Here's how the part is built. I have some questions about the finished solid (model axes, mm). Face numbers are marked on the shaded views. A direction names the side the tool comes from. Round coordinates to 2 decimals unless told otherwise and drop trailing zeros. Loops run counter-clockwise (first coordinate to the right, second up) from the corner with the lowest first, then second, coordinate; pieces in that order, holes last. Notation, with made-up numbers: M 69,11 L 106,11 A19 cw 106,30 Z; hole C -11.5,32.5 d6. An arc over 180 degrees is marked long. Answer as a JSON object with one key per item and string values.
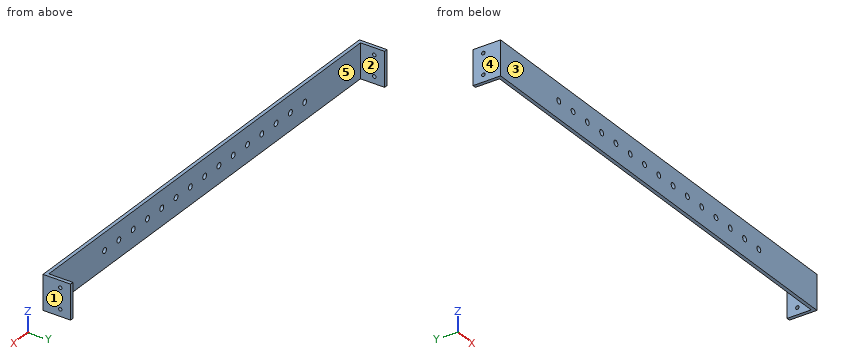
from build123d import *

# Parameters (mm, degrees)
F1_DEPTH      = 25
F2_R          = 4
F3_DEPTH      = 25
F4_R          = 2.5
F5_DEPTH      = 332.001
F5_DEPTH_BACK = 332.001


with BuildPart() as f1:
    # F0 (on Top) → F1 (new body, symmetric)
    with BuildSketch(Plane.XY):
        Polygon((-332, 0), (0, 0), (332, 0), (332, 40), (327, 40), (327, 5), (0, 5), (-327, 5), (-327, 40), (-332, 40), align=None)
    extrude(amount=F1_DEPTH, both=True)

    # F2 (on face) → F3 (cut)
    with BuildSketch(Plane.XZ):
        Circle(F2_R)
        with Locations((30, 0)):
            Circle(F2_R)
        with Locations((60, 0)):
            Circle(F2_R)
        with Locations((90, 0)):
            Circle(F2_R)
        with Locations((120, 0)):
            Circle(F2_R)
        with Locations((150, 0)):
            Circle(F2_R)
        with Locations((180, 0)):
            Circle(F2_R)
        with Locations((210, 0)):
            Circle(F2_R)
        with Locations((-30, 0)):
            Circle(F2_R)
        with Locations((-60, 0)):
            Circle(F2_R)
        with Locations((-90, 0)):
            Circle(F2_R)
        with Locations((-120, 0)):
            Circle(F2_R)
        with Locations((-150, 0)):
            Circle(F2_R)
        with Locations((-180, 0)):
            Circle(F2_R)
        with Locations((-210, 0)):
            Circle(F2_R)
    extrude(amount=-F3_DEPTH, mode=Mode.SUBTRACT)

    # F4 (on Right) → F5 (cut, two sides)
    with BuildSketch(Plane.YZ) as f5_sk:
        with Locations((25, 15)):
            Circle(F4_R)
        with Locations((25, -15)):
            Circle(F4_R)
    extrude(amount=F5_DEPTH, mode=Mode.SUBTRACT)
    extrude(f5_sk.sketch, amount=-F5_DEPTH_BACK, mode=Mode.SUBTRACT)


solid = f1.part
Item 1: On a 3-axis mill with a long thin cutter (end or side, diameter ignored), from which of +Z, -Z, +X, -X, +Y, -Y can I reach the whole of each face in a straight line? I mean the marked faces 1 and 2. Say none if no direction works.
Resolved:
{"face 1": "+Z, -Z, +X, +Y, -Y", "face 2": "+Z, -Z, +Y"}
Item 2: Please list where these lines run through material, in increasing order: probe 1 along X at (y, z) = (19.5, -12.5); probe 2 along Y at (x, z) = (329, -15); probe 3 along Z at (x, y) = (60, 1.5). Write a range as from..to.
Resolved:
{"probe 1": "-332..-327, 327..332", "probe 2": "0..22.5, 27.5..40", "probe 3": "-25..-4, 4..25"}
Item 3: I'm going to push a flat-ended pin straight in: pin 1 Ø25 at (x, z) = (-72, -6.5) entering from +Y. Where does the tip first touch, or does it pass through?
Resolved:
{"pin 1": "y = 5"}
Item 4: I want a section at A-A, the plane x = 16. Please give me the cut outline in (y, z).
Resolved:
{"outline": "M 0,-25 L 5,-25 L 5,25 L 0,25 Z"}
Item 5: If we mould it in two halves opening along X, with no side actions, what happens to the marked faces 3, 4 and 5? For each: pulls with the +X half, pulls with the -X half, needs draft (parallel to the pull), parting line crosses it, or undercut.
Resolved:
{"face 3": "needs draft", "face 4": "pulls with the -X half", "face 5": "undercut"}
